```python
from build123d import *

# Parameters (mm, degrees)
F0_R     = 51
F0_W     = 45
F0_H     = 25
F1_DEPTH = 6
F2_W     = 6
F2_H     = 10
F3_DEPTH = 6
F5_R     = 2
F6_D     = 1.5
F8_SIZE  = 0.5


with BuildPart() as f1:
    # F0 (on Top) → F1 (new body)
    with BuildSketch(Plane.XY):
        Circle(F0_R)
        with Locations((0, -27.5)):
            Rectangle(F0_W, F0_H, mode=Mode.SUBTRACT)
        with BuildLine():
            Line((43.874821937, -10), (-43.874821937, -10))
            ThreePointArc((-43.874821937, -10), (0, 45), (43.874821937, -10))
        make_face(mode=Mode.SUBTRACT)
    extrude(amount=F1_DEPTH)

    # F2 (on face) → F3 (join)
    with BuildSketch(Plane.XY.offset(6)):
        with Locations((-32.5, -15)):
            Rectangle(F2_W, F2_H)
    extrude(amount=F3_DEPTH)

    # F5
    f5_edges = [f1.edges().sort_by_distance(p)[0] for p in [
        (-29.5, -15, 12),
        (-35.5, -15, 12),
    ]]
    fillet(f5_edges, radius=F5_R)

    # F6 (through all)
    with Locations(Plane(origin=(0, -10, 0), x_dir=(-1, 0, 0), z_dir=(0, 1, 0))):
        with Locations((32.5, 9)):
            Hole(F6_D / 2)

    # F7: F1 across plane


with BuildPart() as f1_1:
    add(f1.part)
    add(f1.part.mirror(Plane.YZ))

    # F8
    f8_edges = [f1_1.edges().sort_by_distance(p)[0] for p in [
        (-51, 0, 6),
        (-51, 0, 0),
    ]]
    chamfer(f8_edges, length=F8_SIZE)


solid = f1_1.part
```
The model under review builds one solid part; all positions refer to its coordinate system, in mm. A direction names the side the tool comes from. Round coordinates to 2 decimals unless told otherwise and drop trailing zeros. Loops run counter-clockwise (first coordinate to the right, second up) from the corner with the lowest first, then second, coordinate; pieces in that order, holes last. Notation, with made-up numbers: (43.5, 50) -> (75.5, 50) arc R20 ccw to (75.5, 87) -> close; hole circle Ø8 at (70, 53). An arc over 180 degrees is marked (long way). Answer as a JSON object with one key per item and string values. Group by question number.
1) We need section A-A on x = 0. Write out the cut boundary in (y, z).
2) We need section D-D on x = -12.5. Give the number of separate pieces and of enclosed holes in the cut face, then the cut area to 3 significant figures.
3) For faces 1 (the face through (-22.5, -28, 3)), 2 (the face through (29.5, -15, 8)), 3 (the face through (-35.5, -15, 8)), list the 3-axis set-ups (+Z, -Z, +X, -X, +Y, -Y) from which the entire face can be reached by the end or side of a thin tool; tool diameter is ignored.
4) For pin 1 Ø5 at (x, z) = (-4.5, 4) entering from -Y; pin 2 Ø5 at (y, z) = (-28, 4) entering from +X; pin 3 Ø4 at (x, z) = (12.5, 8.5) entering from -Y; pin 4 Ø6 at (x, z) = (-18.5, 5.5) entering from +Y, all flat-tipped, find the tip position at first contact; note any pin that passes through.
5) We need section B-B on y = 0. Write out the cut boundary in (x, z).
6) We need section C-C on z = 4. Write out the cut boundary in (x, y), then the cut area to 3 significant figures.
7) For line 1 (Y direction, x = 0, z = 2.2); line 2 (Y direction, x = -5.5, z = 5.5); line 3 (Z direction, x = 32.5, y = -16.25), list the stretches that pass through material, from the lowest coordinate up. Write a range as [from, to].
Result set:
{
 "1": {"outline": "(-51, 0.5) -> (-50.5, 0) -> (-40, 0) -> (-40, 6) -> (-50.5, 6) -> (-51, 5.5) -> close; (-15, 0) -> (-10, 0) -> (-10, 6) -> (-15, 6) -> close; (45, 0) -> (50.5, 0) -> (51, 0.5) -> (51, 5.5) -> (50.5, 6) -> (45, 6) -> close"},
 "2": {"separate pieces": "3", "enclosed holes": "0", "area": "123 mm²"},
 "3": {"face 1": "+Z, -Z", "face 2": "+Z, +Y, -Y", "face 3": "+Z, -X, +Y, -Y"},
 "4": {"pin 1": "y = -50.96", "pin 2": "x = 44.17", "pin 3": "through", "pin 4": "y = 48.59"},
 "5": {"outline": "(-51, 0.5) -> (-50.5, 0) -> (-45, 0) -> (-45, 6) -> (-50.5, 6) -> (-51, 5.5) -> close; (45, 0) -> (50.5, 0) -> (51, 0.5) -> (51, 5.5) -> (50.5, 6) -> (45, 6) -> close"},
 "6": {"outline": "circle Ø102 at (0, 0); hole (-43.87, -10) -> (43.87, -10) arc R45 ccw (long way) to start; hole (-22.5, -40) -> (22.5, -40) -> (22.5, -15) -> (-22.5, -15) -> close", "area": "2,970 mm²"},
 "7": {"line 1": "[-51, -40], [-15, -10], [45, 51]", "line 2": "[-50.7, -40], [-15, -10], [44.66, 50.7]", "line 3": "[0, 8.25], [9.75, 12]"}
}
